```python
from build123d import *

# Parameters (mm, degrees)
ESQUISSE2_R             = 1.45
ENL_V_MAT_EXTRU_1_DEPTH = 29.219319623
ESQUISSE3_W             = 10
ESQUISSE3_H             = 10
ENL_V_MAT_EXTRU_2_DEPTH = 4.5
BOSS_EXTRU_1_START      = 4
ESQUISSE4_W             = 8
ESQUISSE4_H             = 8
ESQUISSE4_R             = 2.1
BOSS_EXTRU_1_DEPTH      = 4
ESQUISSE5_R             = 3.45
ENL_V_MAT_EXTRU_3_DEPTH = 29.988445974
CHANFREIN1_SIZE         = 0.5


with BuildPart() as part:
    # Esquisse1 → Révolution1 (revolve)
    with BuildSketch(Plane.XY, mode=Mode.PRIVATE) as r_volution1_sk:
        Polygon((0, 19.8), (0, 2.1), (-6, 2.1), (-6, 8), (-2.5, 8), (-2.5, 19.8), align=None)
    revolve(r_volution1_sk.sketch.rotate(Axis((0, 0, 0), (1, 0, 0)), 90), axis=Axis((0, 0, 0), (1, 0, 0)))

    # Esquisse2 → Enlèv. mat.-Extru.1 (cut, through all)
    with BuildSketch(Plane.ZY.offset(2.5)):
        with Locations((0, 10)):
            Circle(ESQUISSE2_R)
        with Locations((-10, 0)):
            Circle(ESQUISSE2_R)
        with Locations((10, 0)):
            Circle(ESQUISSE2_R)
        with Locations((0, -10)):
            Circle(ESQUISSE2_R)
    extrude(amount=-ENL_V_MAT_EXTRU_1_DEPTH, mode=Mode.SUBTRACT)

    # Esquisse3 → Enlèv. mat.-Extru.2 (cut)
    with BuildSketch(Plane(origin=(0, 0, 0), x_dir=(0, 0, -1), z_dir=(1, 0, 0))):
        Rectangle(ESQUISSE3_W, ESQUISSE3_H)
    extrude(amount=-ENL_V_MAT_EXTRU_2_DEPTH, mode=Mode.SUBTRACT)

    # Esquisse4 → Boss.-Extru.1 (add)
    with BuildSketch(Plane.ZY.offset(6).offset(BOSS_EXTRU_1_START)):
        Rectangle(ESQUISSE4_W, ESQUISSE4_H)
        Circle(ESQUISSE4_R, mode=Mode.SUBTRACT)
    extrude(amount=-BOSS_EXTRU_1_DEPTH)

    # Esquisse5 → Enlèv. mat.-Extru.3 (cut, through all)
    with BuildSketch(Plane.ZY.offset(2.5)):
        with Locations((0, 10)):
            Circle(ESQUISSE5_R)
        with Locations((10, 0)):
            Circle(ESQUISSE5_R)
        with Locations((0, -10)):
            Circle(ESQUISSE5_R)
        with Locations((-10, 0)):
            Circle(ESQUISSE5_R)
    extrude(amount=ENL_V_MAT_EXTRU_3_DEPTH, mode=Mode.SUBTRACT)

    # Chanfrein1
    chanfrein1_edges = [part.edges().sort_by_distance(p)[0] for p in [
        (-8, -4, 4),
        (-8, 4, 4),
        (-8, 4, -4),
        (-8, -4, -4),
    ]]
    chamfer(chanfrein1_edges, length=CHANFREIN1_SIZE)


solid = part.part
```
Check sheet for the modelled part. Datum: model origin and axes. Units: mm. A direction names the side the tool comes from. Give positions to 0.01 mm unless a question says otherwise; leave off trailing zeros. Loops run counter-clockwise (first coordinate to the right, second up) from the corner with the lowest first, then second, coordinate; pieces in that order, holes last. Notation, with made-up numbers: M -15.5,-20.75 L -6.5,-20.75 A22 cw -6.5,17.25 Z; hole C 35.5,14.25 d9. An arc over 180 degrees is marked long. Answer as CSV lines item,"result".
Item 1: Set-up check for faces 4 (the face through (-4.23, 6.55, -0.04)), 5 (the face through (-8, 0, 4)), 6 (the face through (-4.23, 0.04, 6.55)), 7 (the face through (-4.226, 5.62, -5.694)), 8 (the face through (-8, 0, -4)): record each of +Z, -Z, +X, -X, +Y, -Y from which the full face is reachable in a straight line by a thin tool's end or side.
Reply:
face 4,"-X, +Y"
face 5,"+Z, -X, +Y, -Y"
face 6,"+Z, -X"
face 7,"-Z, -X, +Y"
face 8,"-Z, -X, +Y, -Y"
Item 2: Scan lines: L1, parallel to Y at x = -0.6, z = 0; L2, parallel to Y at x = -4.8, z = 0; L3, parallel to X at y = -5.5, z = -1. Record each from-to range of solid material in increasing order.
Reply:
L1,"-19.8 to -11.45, -8.55 to -5, 5 to 8.55, 11.45 to 19.8"
L2,"-6.55 to -2.1, 2.1 to 6.55"
L3,"-6 to 0"
Item 3: Depth check by flat-ended pin: pin 1 Ø3 at (x, z) = (-8, 1.5) entering from +Y; pin 2 Ø5 at (x, y) = (-4, 2) entering from +Z; pin 3 Ø4 at (x, y) = (-7.5, 4) entering from +Z; pin 4 Ø5 at (x, y) = (-5.5, -3) entering from -Z. Enter the tip coordinate at first touch or a pass-through.
Reply:
pin 1,"y = 4"
pin 2,"z = 19.8"
pin 3,"z = 7.54"
pin 4,"z = -7.6"
Item 4: Draft check along Y on faces 1 (the face through (-4.23, -6.55, 0.04)), 2 (the face through (-4.226, 5.694, 5.62)), 3 (the face through (-1.268, 8.584, -0.314)). Enter one of: pulls with the +Y half, pulls with the -Y half, needs draft (parallel to the pull), parting line crosses it, or undercut.
Reply:
face 1,"pulls with the -Y half"
face 2,"pulls with the +Y half"
face 3,"undercut"
Item 5: Sectioned sample at C-C, the plane x = -1.25. Enter the section's corners in (y, z), then the cut area to 3 significant figures.
Reply:
outline,"C 0,0 d39.6; hole C -10,0 d2.9; hole M -5,-5 L 5,-5 L 5,5 L -5,5 Z; hole C 0,-10 d2.9; hole C 0,10 d2.9; hole C 10,0 d2.9"
area,"1,110 mm^2"
Item 6: Sectioned sample at A-A, the plane z = 0. Enter the section's corners in (x, y).
Reply:
outline,"M -10,-4 L -6,-4 L -6,-6.55 L -2.5,-6.55 L -2.5,-8.55 L 0,-8.55 L 0,-5 L -4.5,-5 L -4.5,-2.1 L -10,-2.1 Z; M -10,2.1 L -4.5,2.1 L -4.5,5 L 0,5 L 0,8.55 L -2.5,8.55 L -2.5,6.55 L -6,6.55 L -6,4 L -10,4 Z; M -2.5,-19.8 L 0,-19.8 L 0,-11.45 L -2.5,-11.45 Z; M -2.5,11.45 L 0,11.45 L 0,19.8 L -2.5,19.8 Z"
Item 7: Sectioned sample at B-B, the plane y = -10.5. Enter the section's corners in (x, z), then the cut area to 3 significant figures.
Reply:
outline,"M -2.5,-16.79 L 0,-16.79 L 0,-1.36 L -2.5,-1.36 Z; M -2.5,1.36 L 0,1.36 L 0,16.79 L -2.5,16.79 Z"
area,"77.1 mm^2"
Item 8: Sectioned sample at D-D, the plane x = -8.5. Enter the section's corners in (y, z), then the cut area to 3 significant figures.
Reply:
outline,"M -4,-3.5 L -3.5,-4 L 3.5,-4 L 4,-3.5 L 4,3.5 L 3.5,4 L -3.5,4 L -4,3.5 Z; hole C 0,0 d4.2"
area,"49.6 mm^2"
